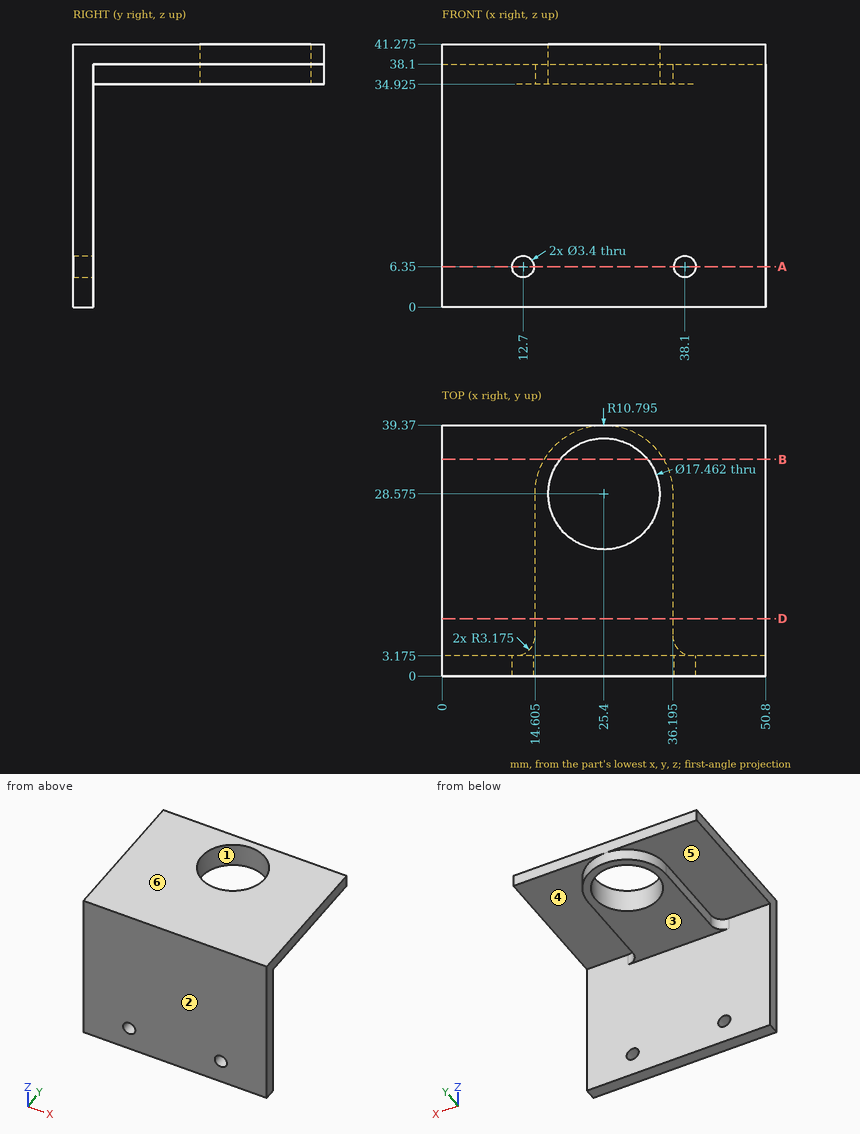
Geometry check sheet. Reference: drawing and pictorial views, mm from the part's lowest x, y, z. A direction names the side the tool comes from. Give positions to 0.01 mm unless a question says otherwise; leave off trailing zeros. Order: outer loops, then holes, each group sorted by start corner. A loop starts at its lowest first (then second) coordinate and runs counter-clockwise, first axis right, second up. Notation, with made-up numbers: M 64.25,52 L 96.25,52 A15 cw 96.25,56 Z; hole C 26,25.5 d10. An arc over 180 degrees is marked long. Return JSON: item names as keys, results as strings. Group by question number.
1) Access from +Z, -Z, +X, -X, +Y, -Y to the whole of each face (thin tool, end or side, straight path). Record for the marked faces 4, 5 and 6.
2) Section check A-A on z = 6.35. Record the cut outline in (x, y) (1 decimal).
3) Go/stop test with flat-tipped pins: pin 1 Ø5.5 at (x, z) = (38.1, 6.35) entering from +Y (1 decimal); pin 2 Ø12 at (x, y) = (32, 33) entering from -Z (1 decimal); pin 3 Ø1 at (y, z) = (20, 36.5) entering from -X (1 decimal). Record where each tip stops, or that it passes through.
4) Scan lines: line 1 (X direction, y = 1.45, z = 6.35); line 2 (Y direction, x = 25.4, z = 39.25); line 3 (Z direction, x = 32, y = 20) (1 decimal). Record each from-to range of solid material in increasing order.
5) Section check B-B on y = 34. Record the cut outline in (x, z) (1 decimal), and give its area (3 significant figures).
6) Section check D-D on y = 9. Record the cut outline in (x, z) (1 decimal), and give its area (3 significant figures).
7) Mould release check, pull along Y, two halves, no side actions. Record for the marked faces 1, 2 and 3: pulls with the +Y half, pulls with the -Y half, needs draft (parallel to the pull), parting line crosses it, or undercut.
Answer block:
{
 "1": {"face 4": "-Z, +X, +Y", "face 5": "-Z, -X, +Y", "face 6": "+Z, +X, -X, +Y, -Y"},
 "2": {"outline": "M 0,0 L 11,0 L 11,3.2 L 0,3.2 Z; M 14.4,0 L 36.4,0 L 36.4,3.2 L 14.4,3.2 Z; M 39.8,0 L 50.8,0 L 50.8,3.2 L 39.8,3.2 Z"},
 "3": {"pin 1": "stops at y = 3.2", "pin 2": "stops at z = 34.9", "pin 3": "stops at x = 14.6"},
 "4": {"line 1": "x = 0 to 11, 14.4 to 36.4, 39.8 to 50.8", "line 2": "y = 0 to 19.84, 37.31 to 39.37", "line 3": "z = 34.9 to 41.3"},
 "5": {"outline": "M 0,38.1 L 16.1,38.1 L 16.1,34.9 L 18.6,34.9 L 18.6,41.3 L 0,41.3 Z; M 32.2,34.9 L 34.7,34.9 L 34.7,38.1 L 50.8,38.1 L 50.8,41.3 L 32.2,41.3 Z", "area": "134 mm^2"},
 "6": {"outline": "M 0,38.1 L 14.6,38.1 L 14.6,34.9 L 36.2,34.9 L 36.2,38.1 L 50.8,38.1 L 50.8,41.3 L 0,41.3 Z", "area": "230 mm^2"},
 "7": {"face 1": "undercut", "face 2": "pulls with the -Y half", "face 3": "needs draft"}
}
